Read the model definition and answer for the solid it produces. Units are mm, in the model's axes. A direction names the side the tool comes from. Coordinates: 2 decimals unless noted, no trailing zeros. Loops run counter-clockwise (first coordinate to the right, second up) from the corner with the lowest first, then second, coordinate; pieces in that order, holes last. Notation, with made-up numbers: (47, -0.75) -> (51, -0.75) arc R31 cw to (51, 27.25) -> close; hole circle Ø7 at (84, 73.25). An arc over 180 degrees is marked (long way). Answer as CSV lines item,"result".
```python
from build123d import *

# Parameters (mm, degrees)
BOSS_EXTRUDE1_DEPTH     = 11.43
SKETCH2_W               = 8.89
SKETCH2_H               = 3.175
BOSS_EXTRUDE2_DEPTH     = 2.54
SKETCH3_R               = 1.524
CUT_EXTRUDE1_DEPTH      = 11.795
CUT_EXTRUDE2_DEPTH      = 1
CUT_EXTRUDE2_DEPTH_BACK = 44.701
CHAMFER1_SIZE           = 1.524


with BuildPart() as part:
    # Sketch1 → Boss-Extrude1 (new body)
    with BuildSketch(Plane.XY):
        with BuildLine():
            Line((-20.079, 0), (-20.079, 1.905))
            Line((-20.079, 1.905), (-31.763, 1.905))
            Line((-31.763, 1.905), (-31.763, -4.445))
            Line((-31.763, -4.445), (-34.811, -4.445))
            Line((-34.811, -4.445), (-34.811, 2.168459549))
            ThreePointArc((-34.811, 2.168459549), (-34.627401057, 3.091473766), (-34.104555503, 3.873967435))
            Line((-34.104555503, 3.873967435), (-33.731967435, 4.246555503))
            ThreePointArc((-33.731967435, 4.246555503), (-32.949473766, 4.769401057), (-32.026459549, 4.953))
            Line((-32.026459549, 4.953), (-19.817153407, 4.953))
            ThreePointArc((-19.817153407, 4.953), (-18.89413919, 4.769401057), (-18.11164552, 4.246555503))
            Line((-18.11164552, 4.246555503), (-17.619534515, 3.754444497))
            ThreePointArc((-17.619534515, 3.754444497), (-16.837040845, 3.231598943), (-15.914026628, 3.048))
            Line((-15.914026628, 3.048), (-5.436586327, 3.048))
            ThreePointArc((-5.436586327, 3.048), (-4.51357211, 3.231598943), (-3.731078441, 3.754444497))
            Line((-3.731078441, 3.754444497), (-1.841967435, 5.643555503))
            ThreePointArc((-1.841967435, 5.643555503), (-1.059473766, 6.166401057), (-0.136459549, 6.35))
            Line((-0.136459549, 6.35), (8.89, 6.35))
            Line((8.89, 6.35), (8.89, 3.175))
            Line((8.89, 3.175), (0, 3.175))
            Line((0, 3.175), (0, 0))
            Line((0, 0), (-20.079, 0))
        make_face()
    extrude(amount=BOSS_EXTRUDE1_DEPTH)

    # Sketch2 → Boss-Extrude2 (add)
    with BuildSketch(Plane.XY.offset(11.43)):
        with Locations((4.445, 1.5875)):
            Rectangle(SKETCH2_W, SKETCH2_H)
    extrude(amount=-BOSS_EXTRUDE2_DEPTH)

    # Sketch3 → Cut-Extrude1 (cut, through all)
    with BuildSketch(Plane(origin=(0, 6.35, 0), x_dir=(1, 0, 0), z_dir=(0, 1, 0))):
        with Locations((4.445, -4.445)):
            Circle(SKETCH3_R)
    extrude(amount=-CUT_EXTRUDE1_DEPTH, mode=Mode.SUBTRACT)

    # Sketch4 → Cut-Extrude2 (cut, two sides)
    with BuildSketch(Plane(origin=(8.89, 0, 0), x_dir=(0, 0, -1), z_dir=(1, 0, 0))) as cut_extrude2_sk:
        with BuildLine():
            Line((-11.43, 3.175), (-11.43, 2.54))
            ThreePointArc((-11.43, 2.54), (-10.314076836, 5.234076836), (-7.62, 6.35))
            Line((-7.62, 6.35), (-11.43, 6.35))
            Line((-11.43, 6.35), (-11.43, 3.175))
        make_face()
        with BuildLine():
            Line((0, 6.35), (-1.27, 6.35))
            ThreePointArc((-1.27, 6.35), (-0.371974388, 5.978025612), (0, 5.08))
            Line((0, 5.08), (0, 6.35))
        make_face()
    extrude(amount=CUT_EXTRUDE2_DEPTH, mode=Mode.SUBTRACT)
    extrude(cut_extrude2_sk.sketch, amount=-CUT_EXTRUDE2_DEPTH_BACK, mode=Mode.SUBTRACT)

    # Chamfer1
    chamfer1_edges = [part.edges().sort_by_distance(p)[0] for p in [
        (2.921, 6.35, 4.445),
    ]]
    chamfer(chamfer1_edges, length=CHAMFER1_SIZE)


solid = part.part
```
Q1. A cutting plane is placed at C-C, the plane x = -4.5. Write down the section's boundary in (y, z).
Results:
outline,"(0, 0) -> (3.24, 0) -> (3.24, 11.37) arc R3.81 ccw to (2.54, 11.43) -> (0, 11.43) -> close"
Q2. Find the intervals of material crossed by probe 1 along Y at (x, z) = (-21, 1.5) (3 decimals); probe 2 along X at (y, z) = (-2.5, 1); probe 3 along Z at (x, y) = (3, 0.25), in increasing order. Write a range as [from, to].
Results:
probe 1,"y = [1.905, 4.953]"
probe 2,"x = [-34.81, -31.76]"
probe 3,"z = [8.89, 11.43]"
Q3. For faces 5 (the face through (-20.079, 1, 6)), 6 (the face through (0, 2, 4)), 7 (the face through (-2.8, 4.686, 5.537)), determine the directions among +Z, -Z, +X, -X, +Y, -Y from which every point of the face is accessible in a straight line to the end or side of a thin tool.
Results:
face 5,"+Z, -Z, -Y"
face 6,"-Z, +X, -Y"
face 7,"+Z, -Z, +Y"
Q4. For a pull along X with two mould halves and no side action, classify faces 1 (the face through (-13, 1, 11.43)), 2 (the face through (-32.962, 4.764, 5.436)), 3 (the face through (-16.849, 3.237, 5.618)), 4 (the face through (5.148, 4.012, 5.797)) as pulls with the +X half, pulls with the -X half, needs draft (parallel to the pull), parting line crosses it, or undercut.
Results:
face 1,"needs draft"
face 2,"pulls with the -X half"
face 3,"undercut"
face 4,"undercut"
Q5. A cutting plane is placed at B-B, the plane y = -2.75. Write down the section's boundary in (x, z).
Results:
outline,"(-34.81, 0) -> (-31.76, 0) -> (-31.76, 11.43) -> (-34.81, 11.43) -> close"
Q6. Given pin 1 Ø5 at (x, z) = (-11.5, 7) entering from +Y; pin 2 Ø6 at (x, z) = (-18.5, 2) entering from +Y; pin 3 Ø1.6 at (y, z) = (2, 3.5) entering from +X, each flat-ended and moving along its own axis, determine where each tip first touches the part or whether it passes through.
Results:
pin 1,"stops at y = 3.05"
pin 2,"stops at y = 4.95"
pin 3,"stops at x = 0"
Q7. A cutting plane is placed at A-A, the plane x = -14. Write down the section's boundary in (y, z).
Results:
outline,"(0, 0) -> (3.05, 0) -> (3.05, 11.4) arc R3.81 ccw to (2.54, 11.43) -> (0, 11.43) -> close"
